from build123d import *

# Parameters (mm, degrees)
F1_DEPTH = 1
F2_DEPTH = 4
F3_SIZE  = 0.5
F5_DEPTH = 10


# Not quite as in the source:
# - a feature names something its author has since deleted; it is built from what else it names


with BuildPart() as f1:
    # F0 (on Front) → F1 (new body)
    with BuildSketch(Plane.XZ):
        with BuildLine():
            ThreePointArc((3, 0), (2.1213203436, 2.1213203436), (0, 3))
            ThreePointArc((0, 3), (-2.1213203436, -2.1213203436), (3, 0))
        make_face()
    extrude(amount=-F1_DEPTH)

    # F0 (on Front) → F2 (join)
    with BuildSketch(Plane.XZ):
        with BuildLine():
            ThreePointArc((0, 3.8), (-2.6870057685, -2.6870057685), (3.8, 0))
            ThreePointArc((3.8, 0), (2.6870057685, 2.6870057685), (0, 3.8))
        make_face()
        with BuildLine():
            ThreePointArc((3, 0), (-2.1213203436, -2.1213203436), (0, 3))
            ThreePointArc((0, 3), (2.1213203436, 2.1213203436), (3, 0))
        make_face(mode=Mode.SUBTRACT)
        with BuildLine():
            ThreePointArc((3, 0), (2.1213203436, 2.1213203436), (0, 3))
            ThreePointArc((0, 3), (-2.1213203436, -2.1213203436), (3, 0))
        make_face()
    extrude(amount=F2_DEPTH)

    # F3
    f3_edges = [f1.edges().sort_by_distance(p)[0] for p in [
        (0, -4, -3.8),
        (0, 0, -3.8),
    ]]
    chamfer(f3_edges, length=F3_SIZE)

    # F4 (on face) → F5 (cut)
    with BuildSketch(Plane(origin=(0, 1, 0), x_dir=(-1, 0, 0), z_dir=(0, 1, 0))):
        with BuildLine():
            Line((-1.6233506232, 3.0850012567), (-1.809656001, 3.3414286104))
            ThreePointArc((-1.809656001, 3.3414286104), (-2.2335839587, 3.0742645786), (-2.6186729953, 2.7536433581))
            Line((-2.6186729953, 2.7536433581), (-2.4323676176, 2.4972160044))
            Line((-2.4323676176, 2.4972160044), (-1.6233506232, 3.0850012567))
        make_face()
        with BuildLine():
            Line((0, 3.45), (0, 3.8))
            ThreePointArc((0, 3.8), (-0.2505451722, 3.7917314141), (-0.5, 3.7669616404))
            Line((-0.5, 3.7669616404), (-0.5, 3.45))
            Line((-0.5, 3.45), (0, 3.45))
        make_face()
        with BuildLine():
            Line((0.5, 3.45), (0.5, 3.7669616404))
            ThreePointArc((0.5, 3.7669616404), (0.2505451722, 3.7917314141), (0, 3.8))
            Line((0, 3.8), (0, 3.45))
            Line((0, 3.45), (0.5, 3.45))
        make_face()
        with BuildLine():
            ThreePointArc((3.4280849175, -1.6395834222), (3.6140147619, -1.1742645786), (3.7371019119, -0.6885269059))
            Line((3.7371019119, -0.6885269059), (3.4356534784, -0.5905803724))
            Line((3.4356534784, -0.5905803724), (3.126636484, -1.5416368887))
            Line((3.126636484, -1.5416368887), (3.4280849175, -1.6395834222))
        make_face()
        with BuildLine():
            ThreePointArc((1.809656001, -3.3414286104), (2.2335839587, -3.0742645786), (2.6186729953, -2.7536433581))
            Line((2.6186729953, -2.7536433581), (2.4323676176, -2.4972160044))
            Line((2.4323676176, -2.4972160044), (1.6233506232, -3.0850012567))
            Line((1.6233506232, -3.0850012567), (1.809656001, -3.3414286104))
        make_face()
        with BuildLine():
            ThreePointArc((-0.5, -3.7669616404), (0, -3.8), (0.5, -3.7669616404))
            Line((0.5, -3.7669616404), (0.5, -3.45))
            Line((0.5, -3.45), (-0.5, -3.45))
            Line((-0.5, -3.45), (-0.5, -3.7669616404))
        make_face()
        with BuildLine():
            ThreePointArc((-2.6186729953, -2.7536433581), (-2.2335839587, -3.0742645786), (-1.809656001, -3.3414286104))
            Line((-1.809656001, -3.3414286104), (-1.6233506232, -3.0850012567))
            Line((-1.6233506232, -3.0850012567), (-2.4323676176, -2.4972160044))
            Line((-2.4323676176, -2.4972160044), (-2.6186729953, -2.7536433581))
        make_face()
        with BuildLine():
            ThreePointArc((-3.7371019119, -0.6885269059), (-3.6140147619, -1.1742645786), (-3.4280849175, -1.6395834222))
            Line((-3.4280849175, -1.6395834222), (-3.126636484, -1.5416368887))
            Line((-3.126636484, -1.5416368887), (-3.4356534784, -0.5905803724))
            Line((-3.4356534784, -0.5905803724), (-3.7371019119, -0.6885269059))
        make_face()
        with BuildLine():
            Line((-3.126636484, 1.5416368887), (-3.4280849175, 1.6395834222))
            ThreePointArc((-3.4280849175, 1.6395834222), (-3.6140147619, 1.1742645786), (-3.7371019119, 0.6885269059))
            Line((-3.7371019119, 0.6885269059), (-3.4356534784, 0.5905803724))
            Line((-3.4356534784, 0.5905803724), (-3.126636484, 1.5416368887))
        make_face()
        with BuildLine():
            Line((3.4356534784, 0.5905803724), (3.7371019119, 0.6885269059))
            ThreePointArc((3.7371019119, 0.6885269059), (3.6140147619, 1.1742645786), (3.4280849175, 1.6395834222))
            Line((3.4280849175, 1.6395834222), (3.126636484, 1.5416368887))
            Line((3.126636484, 1.5416368887), (3.4356534784, 0.5905803724))
        make_face()
        with BuildLine():
            Line((2.4323676176, 2.4972160044), (2.6186729953, 2.7536433581))
            ThreePointArc((2.6186729953, 2.7536433581), (2.2335839587, 3.0742645786), (1.809656001, 3.3414286104))
            Line((1.809656001, 3.3414286104), (1.6233506232, 3.0850012567))
            Line((1.6233506232, 3.0850012567), (2.4323676176, 2.4972160044))
        make_face()
    extrude(amount=-F5_DEPTH, mode=Mode.SUBTRACT)


solid = f1.part
Model file for the job. Use its own axes, mm. A direction names the side the tool comes from. Coordinates: 2 decimals unless noted, no trailing zeros. Write each question's results on one line, items separated by ' | '. Start each with the question number.
1) Mould opens along X. For faces 1 (the face through (3.1, -2, 2.2)), 2 (the face through (-2.03, -1.97, -2.79)), 3 (the face through (0, 1, 0)), 4 (the face through (0, -2, -3.45)) say: pulls with the +X half, pulls with the -X half, needs draft (parallel to the pull), parting line crosses it, or undercut.
2) 3-axis set-ups, long thin cutter, end or side, ignore diameter. For faces 5 (the face through (-2.022, -1.974, 2.795)), 6 (the face through (-3.1, -2, -2.2)), 7 (the face through (0, -2, 3.45)): which of +Z, -Z, +X, -X, +Y, -Y reach the whole face in a straight line?
3) Probe line 1 along Y through (x, z) = (-1.25, 3); line 2 along X through (y, z) = (-3.7, -1); line 3 along Z through (x, y) = (1.5, 0.45). List the from-to ranges inside material, lowest first. Write a range as from..to.
4) Flat gauge pins, fed straight in: P1, Ø3, axis at x = -2, y = -2, coming from the +Z side; P2, Ø0.8, axis at x = 0, y = -2, coming from the +Z side; P3, Ø2, axis at y = -3, z = -3, coming from the +X side. Where does each tip first touch, or does it go through?
Returned:
1) face 1: pulls with the +X half | face 2: undercut | face 3: needs draft | face 4: undercut
2) face 5: +Y, -Y | face 6: -Z, -X, +Y, -Y | face 7: +Z, +Y, -Y
3) line 1: -4..0 | line 2: -3.3..3.3 | line 3: -2.6..2.6
4) P1: z = 3.77 | P2: z = 3.45 | P3: x = 3.23
